from build123d import *

# Parameters (mm, degrees)
SKETCH_W        = 14.8
SKETCH_H        = 10.3
PAD_DEPTH       = 1.5
CHAMFER_SIZE    = 0.5
SKETCH002_W     = 13.8
SKETCH002_H     = 6.2
SKETCH001_W     = 13.8
SKETCH001_H     = 6.28
SKETCH003_W     = 13.2
SKETCH003_H     = 9
PAD001_DEPTH    = 8.7
SKETCH004_W     = 0.4
SKETCH004_H     = 3.7
PAD002_DEPTH    = 6.4
SKETCH005_W     = 1
SKETCH005_H     = 2
POCKET_DEPTH    = 12.601
CHAMFER001_SIZE = 0.5


with BuildPart() as part:
    # Sketch → Pad (new body)
    with BuildSketch(Plane.XY):
        Rectangle(SKETCH_W, SKETCH_H)
    extrude(amount=PAD_DEPTH)

    # Chamfer
    chamfer_edges = [part.edges().sort_by_distance(p)[0] for p in [
        (0, 5.15, 1.5),
        (7.4, 0, 1.5),
        (0, -5.15, 1.5),
        (-7.4, 0, 1.5),
    ]]
    chamfer(chamfer_edges, length=CHAMFER_SIZE)

    # Sketch002 (on DatumPlane) → AdditiveLoft section 0
    with BuildSketch(Plane(origin=(6.523704, 0, 0.21644), x_dir=(0.976296, 0, -0.21644), z_dir=(0.21644, 0, 0.976296))):
        with Locations((-6.9, 0)):
            Rectangle(SKETCH002_W, SKETCH002_H)
    # Sketch001 → AdditiveLoft section 1
    with BuildSketch(Plane.XY):
        Rectangle(SKETCH001_W, SKETCH001_H)
    loft()

    # Sketch003 → Pad001 (join)
    with BuildSketch(Plane.XY):
        Rectangle(SKETCH003_W, SKETCH003_H)
    extrude(amount=-PAD001_DEPTH)

    # Sketch004 (on DatumPlane) → Pad002 (join)
    with BuildSketch(Plane(origin=(0, 0, -8.7), x_dir=(1, 0, 0), z_dir=(0, 0, -1))):
        with Locations((-5, 0)):
            Rectangle(SKETCH004_W, SKETCH004_H)
        Rectangle(SKETCH004_W, SKETCH004_H)
    extrude(amount=PAD002_DEPTH)

    # Sketch005 (on DatumPlane) → Pocket (cut, through all)
    with BuildSketch(Plane(origin=(-5.2, 0, 0), x_dir=(0, -1, 0), z_dir=(-1, 0, 0))):
        with Locations((0, -13)):
            Rectangle(SKETCH005_W, SKETCH005_H)
    extrude(amount=-POCKET_DEPTH, mode=Mode.SUBTRACT)

    # Chamfer001
    chamfer001_edges = [part.edges().sort_by_distance(p)[0] for p in [
        (-5, -1.85, -15.1),
        (0, -1.85, -15.1),
        (0, 1.85, -15.1),
        (-5, 1.85, -15.1),
    ]]
    chamfer(chamfer001_edges, length=CHAMFER001_SIZE)


solid = part.part
Work out the finished part from the listing and answer in its coordinate system (mm). A direction names the side the tool comes from. Round coordinates to 2 decimals unless told otherwise and drop trailing zeros. Write each loop counter-clockwise with the first axis right and the second up, starting at its lowest first coordinate (ties: lowest second). Pieces come first, ordered by that corner, then holes. Notation, with made-up numbers: (-18, 63) - (22, 63) arc R7 cw to (22, 72) - close; hole circle Ø3 at (18.25, 11.5). An arc over 180 degrees is marked (long way). Answer in a Markdown table with one row per item. Add a question column.
1. A cutting plane is placed at B-B, the plane x = 4. Determine the outline of the cut face in (y, z).
2. Given pin 1 (8 mm diameter, centred on x = -4, z = -11.5, fed in from -Y); pin 2 (1 mm diameter, centred on y = 2.5, z = -8.5, fed in from +X); pin 3 (5 mm diameter, centred on x = 5, z = -5.5, fed in from +Y), each flat-ended and moving along its own axis, determine where each tip first touches the part or whether it passes through.
3. A cutting plane is placed at A-A, the plane z = -11. Determine the outline of the cut face in (x, y), and give its area (3 significant figures).
4. A cutting plane is placed at C-C, the plane z = -7. Determine the outline of the cut face in (x, y).
5. The mould has two halves that part along X. Classify faces 1 (the flat face through (-4.8, 0, -11)), 2 (the flat face through (-3.19, 0.03, 2.37)), 3 (the flat face through (-7.4, -0.1, 0.5)): +X half, -X half, draft (parallel to the pull), parting line (faces both ways), or undercut.
6. Find the intervals of material crossed by line 1 along X through (y, z) = (-1.5, -10.5); line 2 along Y through (x, z) = (-5, -2); line 3 along Z through (x, y) = (-5, 3.5), in increasing order. Write a range as from..to.
7. For faces 4 (the flat face through (-6.6, 0, -4)), 5 (the flat face through (0, 4.5, -4)), 6 (the flat face through (0.2, 0, -11)), determine the directions among +Z, -Z, +X, -X, +Y, -Y from which every point of the face is accessible in a straight line to the end or side of a thin tool.
Worked out:
| question | item | result |
|---|---|---|
| 1 | outline | (-5.15, 0) - (-4.5, 0) - (-4.5, -8.7) - (4.5, -8.7) - (4.5, 0) - (5.15, 0) - (5.15, 1) - (4.65, 1.5) - (-4.65, 1.5) - (-5.15, 1) - close |
| 2 | pin 1 | y = -4.5 |
| 2 | pin 2 | x = 6.6 |
| 2 | pin 3 | y = 4.5 |
| 3 | outline | (-5.2, -1.85) - (-4.8, -1.85) - (-4.8, 1.85) - (-5.2, 1.85) - close; (-0.2, -1.85) - (0.2, -1.85) - (0.2, 1.85) - (-0.2, 1.85) - close |
| 3 | area | 2.96 mm^2 |
| 4 | outline | (-6.6, -4.5) - (6.6, -4.5) - (6.6, 4.5) - (-6.6, 4.5) - close |
| 5 | face 1 | undercut |
| 5 | face 2 | +X half |
| 5 | face 3 | -X half |
| 6 | line 1 | -5.2..-4.8, -0.2..0.2 |
| 6 | line 2 | -4.5..4.5 |
| 6 | line 3 | -8.7..1.5 |
| 7 | face 4 | -Z, -X, +Y, -Y |
| 7 | face 5 | -Z, +X, -X, +Y |
| 7 | face 6 | -Z, +X, +Y, -Y |
